Can you work these out from the model? Positions are in its coordinate system, mm. A direction names the side the tool comes from. Coordinates: 2 decimals unless noted, no trailing zeros. Loops run counter-clockwise (first coordinate to the right, second up) from the corner with the lowest first, then second, coordinate; pieces in that order, holes last.
```python
from build123d import *

# Parameters (mm, degrees)
F1_DEPTH = 42.5
F2_W     = 25
F2_H     = 21
F3_DEPTH = 110
F4_W     = 3
F4_H     = 21
F5_DEPTH = 82
F6_W     = 3
F6_H     = 21
F7_DEPTH = 82


with BuildPart() as f1:
    # F0 (on Right) → F1 (new body)
    with BuildSketch(Plane.YZ):
        with BuildLine():
            Line((120, -3), (120, 0))
            Line((120, 0), (10, 0))
            ThreePointArc((10, 0), (2.928932, -2.928932), (0, -10))
            Line((0, -10), (0, -37.5))
            ThreePointArc((0, -37.5), (1.464466, -41.035534), (5, -42.5))
            Line((5, -42.5), (5, -39.5))
            ThreePointArc((5, -39.5), (3.585786, -38.914214), (3, -37.5))
            Line((3, -37.5), (3, -10))
            ThreePointArc((3, -10), (5.050253, -5.050253), (10, -3))
            Line((10, -3), (120, -3))
        make_face()
    extrude(amount=F1_DEPTH)

    # F2 (on face) → F3 (cut)
    with BuildSketch(Plane.XZ):
        with Locations((27, -10.5)):
            Rectangle(F2_W, F2_H)
    extrude(amount=-F3_DEPTH, mode=Mode.SUBTRACT)

    # F4 (on face) → F5 (cut)
    with BuildSketch(Plane.XZ):
        with Locations((13, -10.5)):
            Rectangle(F4_W, F4_H)
    extrude(amount=-F5_DEPTH, mode=Mode.SUBTRACT)

    # F6 (on face) → F7 (cut)
    with BuildSketch(Plane.XZ):
        with Locations((41, -10.5)):
            Rectangle(F6_W, F6_H)
    extrude(amount=-F7_DEPTH, mode=Mode.SUBTRACT)


solid = f1.part
```
(1) If I drill on probe 1 along Z at (x, y) = (41, 115); probe 2 along Y at (x, z) = (40, -29.5); probe 3 along Y at (x, z) = (2, -7), over which ranges is the centre line in solid material (lowest first)?
Check values:
probe 1: z = -3 to 0
probe 2: y = 0 to 3
probe 3: y = 0.46 to 3.68
(2) I want a section at A-A on x = 13. Write out the boundary of the cut face in (y, z).
Check values:
outline: (0, -37.5) arc R5 ccw to (5, -42.5) - (5, -39.5) arc R2 cw to (3, -37.5) - (3, -21) - (0, -21) - close; (82, -3) - (120, -3) - (120, 0) - (82, 0) - close
(3) I want a section at B-B on y = 100.5. Write out the boundary of the cut face in (x, z), then the cut area to 3 significant figures.
Check values:
outline: (0, -3) - (14.5, -3) - (14.5, 0) - (0, 0) - close; (39.5, -3) - (42.5, -3) - (42.5, 0) - (39.5, 0) - close
area: 52.5 mm2
(4) Which directions (+Z, -Z, +X, -X, +Y, -Y) give clear straight access to the entire face, cutting with the end or side of a thin tool? Please do faces 1 (the cylindrical face through (5.7, 5, -5.1)), 2 (the flat face through (11.5, 34.7, -2.8)), 3 (the flat face through (13, 82, -1)).
Check values:
face 1: +X, -X, +Y
face 2: +Z, +X, -Y
face 3: +Z, -Z, +X, -Y
(5) If we mould it in two halves opening along Z, with no side actions, what happens to faces 4 (the flat face through (21, 5, -41)), 5 (the cylindrical face through (5.67, 3.01, -2.85)), 6 (the flat face through (16, 3, -27))? For each: released by +Z, released by -Z, zero draft, split by the parting line, or undercut.
Check values:
face 4: zero draft
face 5: released by +Z
face 6: undercut
(6) I'm going to push flat-ended pins straight in: pin 1 (14 mm diameter, centred on x = 22.5, z = -28, fed in from +Y); pin 2 (2.5 mm diameter, centred on x = 13, z = -2, fed in from -Y); pin 3 (4 mm diameter, centred on x = 34, z = -4.5, fed in from -Y); pin 4 (1.5 mm diameter, centred on y = 100.5, z = -1, fed in from -X). Where does each tip first touch, or does it pass through?
Check values:
pin 1: stops at y = 3
pin 2: stops at y = 82
pin 3: stops at y = 110
pin 4: stops at x = 0
(7) I want a section at C-C on x = 21. Write out the boundary of the cut face in (y, z), then the cut area to 3 significant figures.
Check values:
outline: (0, -37.5) arc R5 ccw to (5, -42.5) - (5, -39.5) arc R2 cw to (3, -37.5) - (3, -21) - (0, -21) - close; (110, -3) - (120, -3) - (120, 0) - (110, 0) - close
area: 96.0 mm2
(8) I want a section at D-D on z = -11.5. Write out the boundary of the cut face in (x, y), then the cut area to 3 significant figures.
Check values:
outline: (0, 0) - (11.5, 0) - (11.5, 3) - (0, 3) - close
area: 34.5 mm2
